For this review, take the finished solid that the model builds, in its own axes (mm). A direction names the side the tool comes from. Coordinates: 2 decimals unless noted, no trailing zeros. Write each loop counter-clockwise with the first axis right and the second up, starting at its lowest first coordinate (ties: lowest second). Pieces come first, ordered by that corner, then holes. Notation, with made-up numbers: (-3, -30) -> (42, -30) arc R24 ccw to (42, -20) -> close; hole circle Ø5 at (35, -25). An arc over 180 degrees is marked (long way). Put each result on its own line as item: value. Start each with the question number.
Item 1: The part is to be moulded in two halves that separate along Z. For faces 4 (the flat face through (32.068, -28.531, -10.466)), 5 (the flat face through (-21.915, -28.531, 10.459)), 6 (the flat face through (0, -29, 33.732)), say which applies: +Z half, -Z half, draft (parallel to the pull), parting line (faces both ways), or undercut.
Item 2: Insertion check: P1, Ø7, axis at y = -28, z = 24, coming from the +X side; P2, Ø1.5, axis at x = -6.5, z = -19, coming from the -Y side; P3, Ø2, axis at y = -9.5, z = -14.5, coming from the +X side. Each pin has a flat end and moves straight along its axis. Give the tip position at first contact, or say it passes through.
Item 3: To check wall thickness, follow L1, parallel to Z at x = -0.5, y = -27; L2, parallel to Y at x = -22, z = 19; L3, parallel to Z at x = 1, y = -16. State the ranges of each line that lie inside material, in increasing order.
Item 4: For faces 1 (the flat face through (13.98, -28.53, -4.49)), 2 (the flat face through (3.175, -29, 24)), 3 (the flat face through (24.13, -28.53, -4.5)), list the 3-axis set-ups (+Z, -Z, +X, -X, +Y, -Y) from which the entire face can be reached by the end or side of a thin tool; tool diameter is ignored.
Item 5: Consider section A-A on z = -12. Give the boundary of the cut face in (x, y), and give its area (3 significant figures).
Item 6: Consider section D-D on z = 0. Give the boundary of the cut face in (x, y), and give its area (3 significant figures).
Item 7: Consider section C-C on y = 6.5. Give the boundary of the cut face in (x, z), and give its area (3 significant figures).
Item 8: Consider section B-B on x = -2. Give the boundary of the cut face in (y, z), and give its area (3 significant figures).
```python
from build123d import *

# Parameters (mm, degrees)
F0_R     = 33.732281
F1_DEPTH = 25.4
F2_W     = 6.35
F2_H     = 19.05
F3_DEPTH = 6.35


with BuildPart() as f1:
    # F0 (on Front) → F1 (new body, symmetric)
    with BuildSketch(Plane.XZ):
        Circle(F0_R)
    extrude(amount=F1_DEPTH, both=True)

    # F2 (on face) → F3 (join)
    with BuildSketch(Plane.XZ.offset(25.4)):
        with Locations((0, 24.207281)):
            Rectangle(F2_W, F2_H)
        Polygon((-11.198657, 10.011996), (-6.061399, 13.744433), (-17.258708, 29.156206), (-22.395966, 25.42377), align=None)
        Polygon((-14.944808, 1.51747), (-12.98255, 7.556679), (-31.100176, 13.443452), (-33.062434, 7.404244), align=None)
        Polygon((-12.98255, -7.556679), (-14.944808, -1.51747), (-33.062434, -7.404244), (-31.100176, -13.443452), align=None)
        Polygon((-6.061399, -13.744433), (-11.198657, -10.011996), (-22.395966, -25.42377), (-17.258708, -29.156206), align=None)
        with Locations((0, -24.207281)):
            Rectangle(F2_W, F2_H)
        Polygon((11.198657, -10.011996), (6.061399, -13.744433), (17.258708, -29.156206), (22.395966, -25.42377), align=None)
        Polygon((14.944808, -1.51747), (12.98255, -7.556679), (31.100176, -13.443452), (33.062434, -7.404244), align=None)
        Polygon((12.98255, 7.556679), (14.944808, 1.51747), (33.062434, 7.404244), (31.100176, 13.443452), align=None)
        Polygon((6.061399, 13.744433), (11.198657, 10.011996), (22.395966, 25.42377), (17.258708, 29.156206), align=None)
    extrude(amount=F3_DEPTH)


solid = f1.part
```
Return value:
1. face 4: -Z half
1. face 5: undercut
1. face 6: +Z half
2. P1: x = 25.86
2. P2: y = -25.4
2. P3: x = 30.91
3. L1: -33.73 to -14.68, 14.68 to 33.73
3. L2: -25.4 to 25.4
3. L3: -33.72 to 33.72
4. face 1: -Y
4. face 2: +Z, -Z, -Y
4. face 3: +X, -Y
5. outline: (-31.57, -31.75) -> (-26.66, -31.75) -> (-26.66, -25.4) -> (-12.64, -25.4) -> (-12.64, -31.75) -> (-8.46, -31.75) -> (-8.46, -25.4) -> (8.46, -25.4) -> (8.46, -31.75) -> (12.64, -31.75) -> (12.64, -25.4) -> (26.66, -25.4) -> (26.66, -31.75) -> (31.57, -31.75) -> (31.57, -25.4) -> (31.53, -25.4) -> (31.53, 25.4) -> (-31.53, 25.4) -> (-31.53, -25.4) -> (-31.57, -25.4) -> close
5. area: 3,320 mm^2
6. outline: (-33.73, -25.4) -> (33.73, -25.4) -> (33.73, 25.4) -> (-33.73, 25.4) -> close
6. area: 3,430 mm^2
7. outline: circle Ø67.46 at (0, 0)
7. area: 3,570 mm^2
8. outline: (-31.75, -33.73) -> (-25.4, -33.73) -> (-25.4, -33.67) -> (25.4, -33.67) -> (25.4, 33.67) -> (-25.4, 33.67) -> (-25.4, 33.73) -> (-31.75, 33.73) -> (-31.75, 14.68) -> (-25.4, 14.68) -> (-25.4, -14.68) -> (-31.75, -14.68) -> close
8. area: 3,660 mm^2
